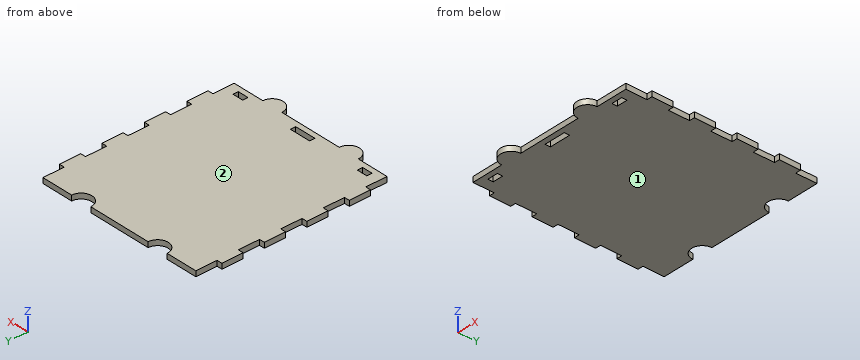
```python
from build123d import *

# Parameters (mm, degrees)
SKETCH1_W           = 10
SKETCH1_H           = 2.5
SKETCH1_W_2         = 5
BOSS_EXTRUDE1_DEPTH = 2.5


with BuildPart() as part:
    # Sketch1 → Boss-Extrude1 (new body)
    with BuildSketch(Plane.XY):
        with BuildLine():
            Line((42.5, 60), (42.5, 50))
            Line((42.5, 50), (40, 50))
            Line((40, 50), (40, 40))
            Line((40, 40), (42.5, 40))
            Line((42.5, 40), (42.5, 30))
            Line((42.5, 30), (40, 30))
            Line((40, 30), (40, 20))
            Line((40, 20), (42.5, 20))
            Line((42.5, 20), (42.5, 10))
            Line((42.5, 10), (40, 10))
            Line((40, 10), (40, 0))
            Line((40, 0), (25, 0))
            ThreePointArc((25, 0), (20, -5), (15, 0))
            Line((15, 0), (-15, 0))
            ThreePointArc((-15, 0), (-20, -5), (-25, 0))
            Line((-25, 0), (-40, 0))
            Line((-40, 0), (-40, 10))
            Line((-40, 10), (-42.5, 10))
            Line((-42.5, 10), (-42.5, 20))
            Line((-42.5, 20), (-40, 20))
            Line((-40, 20), (-40, 30))
            Line((-40, 30), (-42.5, 30))
            Line((-42.5, 30), (-42.5, 40))
            Line((-42.5, 40), (-40, 40))
            Line((-40, 40), (-40, 50))
            Line((-40, 50), (-42.5, 50))
            Line((-42.5, 50), (-42.5, 60))
            Line((-42.5, 60), (-40, 60))
            Line((-40, 60), (-40, 70))
            Line((-40, 70), (-42.5, 70))
            Line((-42.5, 70), (-42.5, 80))
            Line((-42.5, 80), (-40, 80))
            Line((-40, 80), (-40, 90))
            Line((-40, 90), (-25, 90))
            ThreePointArc((-25, 90), (-20, 85), (-15, 90))
            Line((-15, 90), (15, 90))
            ThreePointArc((15, 90), (20, 85), (25, 90))
            Line((25, 90), (40, 90))
            Line((40, 90), (40, 80))
            Line((40, 80), (42.5, 80))
            Line((42.5, 80), (42.5, 70))
            Line((42.5, 70), (40, 70))
            Line((40, 70), (40, 60))
            Line((40, 60), (42.5, 60))
        make_face()
        with Locations((0, 3.75)):
            Rectangle(SKETCH1_W, SKETCH1_H, mode=Mode.SUBTRACT)
        with Locations((32.5, 3.75)):
            Rectangle(SKETCH1_W_2, SKETCH1_H, mode=Mode.SUBTRACT)
        with Locations((-32.5, 3.75)):
            Rectangle(SKETCH1_W_2, SKETCH1_H, mode=Mode.SUBTRACT)
    extrude(amount=BOSS_EXTRUDE1_DEPTH)


solid = part.part
```
CAD build for the part. Positions are in the model's coordinates, mm. Face numbers are marked on the shaded views. Round coordinates to 2 decimals unless told otherwise and drop trailing zeros. Order: outer loops, then holes, each group sorted by start corner. A loop starts at its lowest first (then second) coordinate and runs counter-clockwise, first axis right, second up.
Q1. Drop flat-ended pins along their axis: pin 1 (0.8 mm diameter, centred on y = 83.5, z = 1.5, fed in from -X); pin 2 (1.2 mm diameter, centred on x = -42, z = 1, fed in from -Y); pin 3 (0.8 mm diameter, centred on y = 4, z = 1.5, fed in from +X). Give the stop position or say it passes through.
Q2. Slice it at D-D (x = -21). Write the cut outline in (y, z).
Q3. Slice it at C-C (y = 27). Write the cut outline in (x, z).
Q4. Two-plate mould, pull along Z, no slides. Class the marked faces 1 and 2: pulls with the +Z half, pulls with the -Z half, needs draft (parallel to the pull), parting line crosses it, or undercut.
Q5. Slice it at B-B (z = 0.45). State how many separate pieces and enclosed holes the cut face has, and give its area (3 significant figures).
Q6. Wall check: L1, parallel to X at y = 3, z = 2.1; L2, parallel to Y at x = 3.5, z = 1.3; L3, parallel to Y at x = 20.5, z = 0.2. Give the ranges that are in metal, low to high.
Q7. Slice it at A-A (x = 3). Write the cut outline in (y, z), and give its area (3 significant figures).
Results below:
1. pin 1: stops at x = -40
1. pin 2: stops at y = 10
1. pin 3: stops at x = 40
2. outline: (-4.9, 0) - (85.1, 0) - (85.1, 2.5) - (-4.9, 2.5) - close
3. outline: (-40, 0) - (40, 0) - (40, 2.5) - (-40, 2.5) - close
4. face 1: pulls with the -Z half
4. face 2: pulls with the +Z half
5. separate pieces: 1
5. enclosed holes: 3
5. area: 7,350 mm2
6. L1: x = -40 to -35, -30 to -5, 5 to 30, 35 to 40
6. L2: y = 0 to 2.5, 5 to 90
6. L3: y = -4.97 to 85.03
7. outline: (0, 0) - (2.5, 0) - (2.5, 2.5) - (0, 2.5) - close; (5, 0) - (90, 0) - (90, 2.5) - (5, 2.5) - close
7. area: 219 mm2
